The model under review builds one solid part; all positions refer to its coordinate system, in mm. Round coordinates to 2 decimals unless told otherwise and drop trailing zeros. Write each loop counter-clockwise with the first axis right and the second up, starting at its lowest first coordinate (ties: lowest second). Pieces come first, ordered by that corner, then holes. Notation, with made-up numbers: (76.25, 86) -> (133.25, 86) arc R21 cw to (133.25, 123) -> close; hole circle Ø9 at (57.25, -21). An arc over 180 degrees is marked (long way). Use CSV: the item, a comma, the result in double quotes. Start each with the question number.
1) For pin 1 Ø22.5 at (x, y) = (55.69, -8.96) entering from -Z; pin 2 Ø1.8 at (x, z) = (17, 1.5) entering from +Y; pin 3 Ø1.1 at (x, z) = (-60.5, 1) entering from +Y, all flat-tipped, find the tip position at first contact; note any pin that passes through.
2) Take a section at B-B, the plane z = 1. State how many separate pieces and enclosed holes the cut face has, then the cut area to 3 significant figures.
3) Wall thickness on probe 1 along X at (y, z) = (30, 2); probe 2 along X at (y, z) = (21.5, 0.45); probe 3 along X at (y, z) = (41, 2.2): over which ranges is each line inside the solid? List them lowest first. Write a range as [from, to].
4) Take a section at A-A, the plane x = 61. Give the boundary of the cut face in (y, z).
5) Take a section at C-C, the plane x = 6. Give the boundary of the cut face in (y, z), then the cut area to 3 significant figures.
6) Take a section at D-D, the plane x = 42.5. Give the boundary of the cut face in (y, z), then the cut area to 3 significant figures.
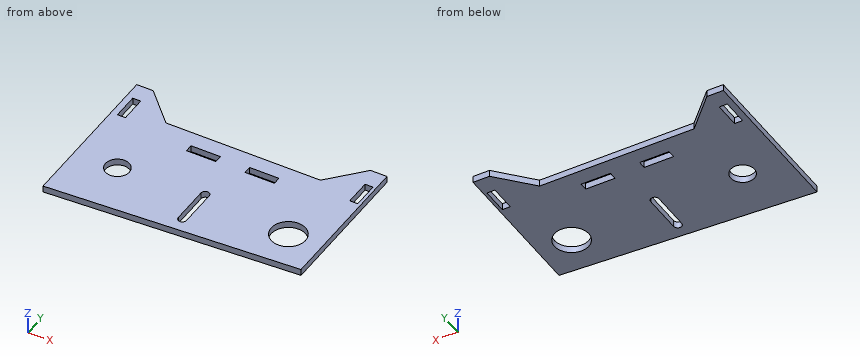
from build123d import *

# Parameters (mm, degrees)
SKETCH2_R           = 9.7
SKETCH2_R_2         = 6.75
SKETCH2_W           = 4.5
SKETCH2_H           = 14.8
SKETCH2_W_2         = 16.6
SKETCH2_H_2         = 4.4
BOSS_EXTRUDE1_DEPTH = 3.7


with BuildPart() as part:
    # Sketch2 → Boss-Extrude1 (new body)
    with BuildSketch(Plane.XY):
        Polygon((-66.408376963, -37.473298429), (-66.408376963, 53.126701571), (-57.108376963, 53.126701571), (-39.206701064, 34.826701571), (48.193298936, 34.826701571), (65.490462758, 53.699118578), (74.790462758, 53.699118578), (74.790462758, -29.400881422), align=None)
        with Locations((55.690462758, -8.957731732)):
            Circle(SKETCH2_R, mode=Mode.SUBTRACT)
        with Locations((-42.158376963, -6.98947646)):
            Circle(SKETCH2_R_2, mode=Mode.SUBTRACT)
        with Locations((-60.558376963, 35.726701571)):
            Rectangle(SKETCH2_W, SKETCH2_H, mode=Mode.SUBTRACT)
        with Locations((70.815419874, 35.726701571)):
            Rectangle(SKETCH2_W, SKETCH2_H, mode=Mode.SUBTRACT)
        with Locations((-11.433419848, 23.626701571)):
            Rectangle(SKETCH2_W_2, SKETCH2_H_2, mode=Mode.SUBTRACT)
        with Locations((21.690462758, 23.626701571)):
            Rectangle(SKETCH2_W_2, SKETCH2_H_2, mode=Mode.SUBTRACT)
        with BuildLine():
            Line((7.428521455, -3.001867406), (7.428521455, -25.037089926))
            ThreePointArc((7.428521455, -25.037089926), (5.128521455, -27.337089926), (2.828521455, -25.037089926))
            Line((2.828521455, -25.037089926), (2.828521455, -3.001867406))
            ThreePointArc((2.828521455, -3.001867406), (5.128521455, -0.701867406), (7.428521455, -3.001867406))
        make_face(mode=Mode.SUBTRACT)
    extrude(amount=BOSS_EXTRUDE1_DEPTH)


solid = part.part
Values found:
1,pin 1,"z = 0"
1,pin 2,"y = 34.83"
1,pin 3,"y = 53.13"
2,separate pieces,"1"
2,enclosed holes,"7"
2,area,"9,480 mm²"
3,probe 1,"[-66.41, -62.81], [-58.31, 68.57], [73.07, 74.79]"
3,probe 2,"[-66.41, -19.73], [-3.13, 13.39], [29.99, 74.79]"
3,probe 3,"[-66.41, -62.81], [-58.31, -45.25], [53.85, 68.57], [73.07, 74.79]"
4,outline,"(-30.19, 0) -> (-17.08, 0) -> (-17.08, 3.7) -> (-30.19, 3.7) -> close; (-0.84, 0) -> (48.8, 0) -> (48.8, 3.7) -> (-0.84, 3.7) -> close"
5,outline,"(-33.33, 0) -> (-27.17, 0) -> (-27.17, 3.7) -> (-33.33, 3.7) -> close; (-0.87, 0) -> (34.83, 0) -> (34.83, 3.7) -> (-0.87, 3.7) -> close"
5,area,"155 mm²"
6,outline,"(-31.25, 0) -> (34.83, 0) -> (34.83, 3.7) -> (-31.25, 3.7) -> close"
6,area,"244 mm²"
